from build123d import *

# Parameters (mm, degrees)
F0_W     = 25.4
F0_H     = 7.634085685
F1_DEPTH = 5.08
F2_T     = -2.54


with BuildPart() as f1:
    # F0 (on Top) → F1 (new body)
    with BuildSketch(Plane.XY):
        Polygon((-7.7176965407, 45.0293049932), (-58.5176965407, 45.0293049932), (-58.5176965407, -31.1706950068), (-45.8176965407, -31.1706950068), (-20.4176965407, -31.1706950068), (-7.7176965407, -31.1706950068), align=None)
        with Locations((-33.1176965407, -34.9877378494)):
            Rectangle(F0_W, F0_H)
    extrude(amount=F1_DEPTH)

    # F2
    f2_openings = [f1.faces().sort_by_distance(p)[0] for p in [
        (-33.117697, 4.929742, 5.08),
    ]]
    offset(amount=F2_T, openings=f2_openings, kind=Kind.INTERSECTION)


solid = f1.part
Input: part model. Units: mm. Frame: model coordinates. A direction names the side the tool comes from. Give positions to 0.01 mm unless a question says otherwise; leave off trailing zeros. Write each loop counter-clockwise with the first axis right and the second up, starting at its lowest first coordinate (ties: lowest second). Pieces come first, ordered by that corner, then holes. Notation, with made-up numbers: (86.25, 21) -> (142.25, 21) arc R24 cw to (142.25, 45) -> close; hole circle Ø10 at (13, 86.25). An arc over 180 degrees is marked (long way). Use one line per item in the form item = value. Start each with the question number.
1) Set-up query: faces 1 (the flat face through (-17, -28.631, 4)), 2 (the flat face through (-58.518, 7, 3)), 3 (the flat face through (-20.418, -35, 3)), 4 (the flat face through (-45.818, -35, 3)), 5 (the flat face through (-7.718, 6, 3)). Return all of +Z, -Z, +X, -X, +Y, -Y with unobstructed straight access to the full face (end or side cutting, diameter ignored); none if empty.
2) Section query A-A on z = 3.65. Return the cut outline in (x, y), then the cut area to 3 significant figures.
3) Section query B-B on y = -23.5. Return the cut outline in (x, z).
4) Pin query (flat end, axial travel): pin 1 (1.5 mm diameter, centred on y = -34, z = 3, fed in from +X); pin 2 (1.5 mm diameter, centred on y = -34.5, z = 2, fed in from -X); pin 3 (1.5 mm diameter, centred on x = -41.5, y = 29.5, fed in from +Z); pin 4 (2 mm diameter, centred on y = -32, z = 4, fed in from +X). Return the tip coordinate at first contact, or that it passes through.
5) Ray query, probe 1 along X at (y, z) = (25, 3.5); probe 2 along X at (y, z) = (-29.5, 3.9); probe 3 along Y at (x, z) = (-14.5, 2.65). Return the intervals inside material, ascending. Write a range as from..to.
6) Section query C-C on x = -51.5. Return the cut outline in (y, z).
Outcome:
q1.face_1 = +Z
q1.face_2 = +Z, -Z, -X, +Y, -Y
q1.face_3 = +Z, -Z, +X, -Y
q1.face_4 = +Z, -Z, -X, -Y
q1.face_5 = +Z, -Z, +X, +Y, -Y
q2.outline = (-58.52, -31.17) -> (-45.82, -31.17) -> (-45.82, -38.8) -> (-20.42, -38.8) -> (-20.42, -31.17) -> (-7.72, -31.17) -> (-7.72, 45.03) -> (-58.52, 45.03) -> close; hole (-55.98, -28.63) -> (-43.28, -28.63) -> (-43.28, -36.26) -> (-22.96, -36.26) -> (-22.96, -28.63) -> (-10.26, -28.63) -> (-10.26, 42.49) -> (-55.98, 42.49) -> close
q2.area = 658 mm^2
q3.outline = (-58.52, 0) -> (-7.72, 0) -> (-7.72, 5.08) -> (-10.26, 5.08) -> (-10.26, 2.54) -> (-55.98, 2.54) -> (-55.98, 5.08) -> (-58.52, 5.08) -> close
q4.pin_1 = -20.42
q4.pin_2 = -45.82
q4.pin_3 = 2.54
q4.pin_4 = -7.72
q5.probe_1 = -58.52..-55.98, -10.26..-7.72
q5.probe_2 = -58.52..-43.28, -22.96..-7.72
q5.probe_3 = -31.17..-28.63, 42.49..45.03
q6.outline = (-31.17, 0) -> (45.03, 0) -> (45.03, 5.08) -> (42.49, 5.08) -> (42.49, 2.54) -> (-28.63, 2.54) -> (-28.63, 5.08) -> (-31.17, 5.08) -> close
